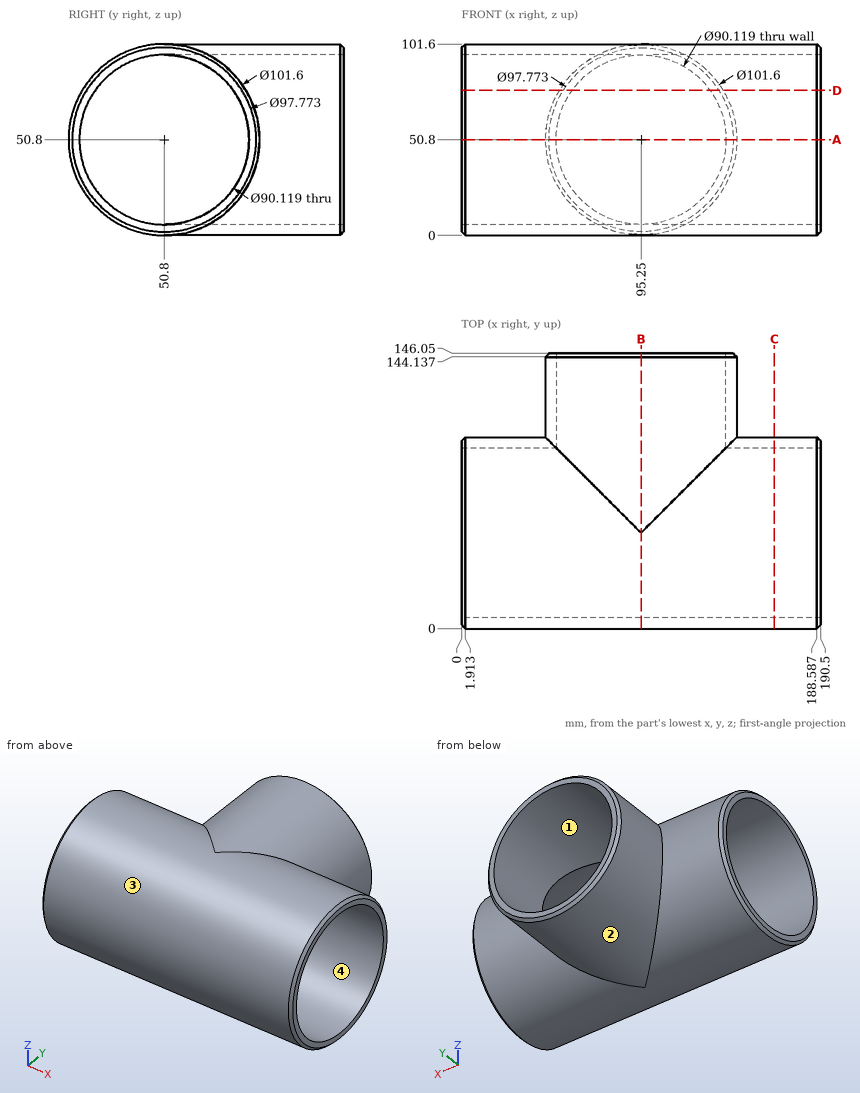
Study the drawing (mm; zero at the part's minimum x, y, z) and answer. A direction names the side the tool comes from. Give positions to 0.01 mm unless a question says otherwise; leave off trailing zeros. Order: outer loops, then holes, each group sorted by start corner. A loop starts at its lowest first (then second) coordinate and runs counter-clockwise, first axis right, second up. Notation, with made-up numbers: (-1, 81) - (48, 81) arc R31 cw to (48, 116) - close; hole circle Ø2 at (24, -16.5). An arc over 180 degrees is marked (long way). Use one line per item in the form item = value. Start each with the question number.
(1) The mould has two halves that part along X. Classify the marked faces 1 and 2: released by +X, released by -X, zero draft, split by the parting line, or undercut.
(2) A cutting plane is placed at A-A, the plane z = 50.8. Write down the section's boundary in (x, y).
(3) Consider line 1 (Z direction, x = 94, y = 50.8); line 2 (Z direction, x = 63, y = 50); line 3 (X direction, y = 121, z = 51.5) (1 decimal). Determine where each line is inside the solid, lowest interval first. Write a range as from..to.
(4) For the marked faces 3 and 4, determine the directions among +Z, -Z, +X, -X, +Y, -Y from which every point of the face is accessible in a straight line to the end or side of a thin tool.
(5) Flat-ended cylindrical pins translate along their axes: pin 1 Ø8 at (y, z) = (23, 79.5) entering from +X; pin 2 Ø6 at (x, y) = (34, 100) entering from -Z (1 decimal); pin 3 Ø8 at (y, z) = (123.5, 81) entering from +X; pin 4 Ø1.5 at (x, y) = (109.5, 120) entering from -Z. Find the tip coordinate at first contact, or state that the pin passes through.
(6) A cutting plane is placed at B-B, the plane x = 95.25. Write down the section's boundary in (y, z).
(7) A cutting plane is placed at D-D, the plane z = 77. State how many separate pieces and enclosed holes the cut face has, then the cut area to 3 significant figures.
(8) A cutting plane is placed at C-C, the plane x = 166. Write down the section's boundary in (y, z).
Ans:
q1.face_1 = undercut
q1.face_2 = split by the parting line
q2.outline = (0, 1.91) - (1.91, 0) - (188.59, 0) - (190.5, 1.91) - (190.5, 5.74) - (0, 5.74) - close; (0, 95.86) - (50.19, 95.86) - (50.19, 146.05) - (46.36, 146.05) - (44.45, 144.14) - (44.45, 101.6) - (1.91, 101.6) - (0, 99.69) - close; (140.31, 95.86) - (190.5, 95.86) - (190.5, 99.69) - (188.59, 101.6) - (146.05, 101.6) - (146.05, 144.14) - (144.14, 146.05) - (140.31, 146.05) - close
q3.line_1 = 0..5.74, 95.86..101.6
q3.line_2 = 0.01..5.75, 95.85..101.59
q3.line_3 = 44.5..50.2, 140.3..146
q4.face_3 = none
q4.face_4 = +X, -X
q5.pin_1 = through
q5.pin_2 = 29.7
q5.pin_3 = 138.77
q5.pin_4 = 1.83
q6.outline = (50.8, 0) - (144.14, 0) - (146.05, 1.91) - (146.05, 5.74) - (50.8, 5.74) arc R45.06 cw to (50.8, 95.86) - (146.05, 95.86) - (146.05, 99.69) - (144.14, 101.6) - (50.8, 101.6) arc R50.8 ccw to start
q7.separate_pieces = 3
q7.enclosed_holes = 0
q7.area = 2,810 mm^2
q8.outline = circle Ø101.6 at (50.8, 50.8); hole circle Ø90.12 at (50.8, 50.8)
